Model file for the job. Use its own axes, mm. A direction names the side the tool comes from. Coordinates: 2 decimals unless noted, no trailing zeros. Loops run counter-clockwise (first coordinate to the right, second up) from the corner with the lowest first, then second, coordinate; pieces in that order, holes last. Notation, with made-up numbers: (35.25, 21.25) -> (61.25, 21.25) arc R28 ccw to (61.25, 50.25) -> close; hole circle Ø1 at (-18, 25). An arc over 180 degrees is marked (long way). Use one line per item in the form item = value.
```python
from build123d import *

# Parameters (mm, degrees)
PAD_DEPTH               = 1
PAD001_DEPTH            = 3
PAD002_DEPTH            = 5
PAD_MIRRORED_2_DEPTH    = 1
PAD001_MIRRORED_2_DEPTH = 3
PAD002_MIRRORED_2_DEPTH = 5


with BuildPart() as part:
    # Sketch → Pad (new body)
    with BuildSketch(Plane.XY):
        with BuildLine():
            Line((0, 0), (19.5, 0))
            Line((19.5, 0), (19.5, 28.5))
            Line((19.5, 28.5), (0, 28.5))
            Line((0, 28.5), (0, 23.2))
            ThreePointArc((0, 18.8), (2.2, 21), (0, 23.2))
            Line((0, 18.8), (0, 0))
        make_face()
    pad = extrude(amount=PAD_DEPTH)

    # Sketch001 → Pad001 (join)
    with BuildSketch(Plane.XY):
        with BuildLine():
            ThreePointArc((0, 18.8), (2.2, 21), (0, 23.2))
            Line((0, 23.2), (0, 26.2))
            ThreePointArc((0, 15.8), (5.2, 21), (0, 26.2))
            Line((0, 18.8), (0, 15.8))
        make_face()
    pad001 = extrude(amount=PAD001_DEPTH)

    # Sketch002 → Pad002 (join)
    with BuildSketch(Plane.XY):
        with BuildLine():
            Line((19.5, 0), (19.5, 28.5))
            Line((19.5, 28.5), (0, 28.5))
            Line((0, 28.5), (0, 31.5))
            Line((0, 31.5), (19.5, 31.5))
            ThreePointArc((22.5, 28.5), (21.62132, 30.62132), (19.5, 31.5))
            Line((22.5, 0), (22.5, 28.5))
            Line((19.5, 0), (22.5, 0))
        make_face()
    pad002 = extrude(amount=PAD002_DEPTH)

    # Sketch Mirrored 2 → Pad Mirrored 2 (add)
    with BuildSketch(Plane(origin=(0, 0, 0), x_dir=(-1, 0, 0), z_dir=(0, 0, -1))):
        with BuildLine():
            Line((0, 0), (19.5, 0))
            Line((19.5, 0), (19.5, 28.5))
            Line((19.5, 28.5), (0, 28.5))
            Line((0, 28.5), (0, 23.2))
            ThreePointArc((0, 18.8), (2.2, 21), (0, 23.2))
            Line((0, 18.8), (0, 0))
        make_face()
    pad_mirrored_2 = extrude(amount=-PAD_MIRRORED_2_DEPTH)

    # Sketch001 Mirrored 2 → Pad001 Mirrored 2 (add)
    with BuildSketch(Plane(origin=(0, 0, 0), x_dir=(-1, 0, 0), z_dir=(0, 0, -1))):
        with BuildLine():
            ThreePointArc((0, 18.8), (2.2, 21), (0, 23.2))
            Line((0, 23.2), (0, 26.2))
            ThreePointArc((0, 15.8), (5.2, 21), (0, 26.2))
            Line((0, 18.8), (0, 15.8))
        make_face()
    pad001_mirrored_2 = extrude(amount=-PAD001_MIRRORED_2_DEPTH)

    # Sketch002 Mirrored 2 → Pad002 Mirrored 2 (add)
    with BuildSketch(Plane(origin=(0, 0, 0), x_dir=(-1, 0, 0), z_dir=(0, 0, -1))):
        with BuildLine():
            Line((19.5, 0), (19.5, 28.5))
            Line((19.5, 28.5), (0, 28.5))
            Line((0, 28.5), (0, 31.5))
            Line((0, 31.5), (19.5, 31.5))
            ThreePointArc((22.5, 28.5), (21.62132, 30.62132), (19.5, 31.5))
            Line((22.5, 0), (22.5, 28.5))
            Line((19.5, 0), (22.5, 0))
        make_face()
    pad002_mirrored_2 = extrude(amount=-PAD002_MIRRORED_2_DEPTH)

    # Mirrored001: Pad, Pad001, Pad002, Pad Mirrored 2, Pad001 Mirrored 2, Pad002 Mirrored 2 across Sketch H_Axis
    add(pad.mirror(Plane.ZX))
    add(pad001.mirror(Plane.ZX))
    add(pad002.mirror(Plane.ZX))
    add(pad_mirrored_2.mirror(Plane.ZX))
    add(pad001_mirrored_2.mirror(Plane.ZX))
    add(pad002_mirrored_2.mirror(Plane.ZX))


solid = part.part
```
Q1. Wall check: line 1 along X through (y, z) = (-21, 1.25); line 2 along X through (y, z) = (14, 1.7); line 3 along Y through (x, z) = (-6, 2.05). Give the ranges that are in metal, low to high.
Result:
line_1 = -22.5 to -19.5, -5.2 to -2.2, 2.2 to 5.2, 19.5 to 22.5
line_2 = -22.5 to -19.5, 19.5 to 22.5
line_3 = -31.5 to -28.5, 28.5 to 31.5
Q2. Band-saw the part on D-D, the plane z = 3.95. Write the cut outline in (x, y).
Result:
outline = (-22.5, -28.5) arc R3 ccw to (-19.5, -31.5) -> (19.5, -31.5) arc R3 ccw to (22.5, -28.5) -> (22.5, 28.5) arc R3 ccw to (19.5, 31.5) -> (-19.5, 31.5) arc R3 ccw to (-22.5, 28.5) -> close; hole (-19.5, -28.5) -> (19.5, -28.5) -> (19.5, 28.5) -> (-19.5, 28.5) -> close
Q3. Band-saw the part on C-C, the plane y = 21. Write the cut outline in (x, z).
Result:
outline = (-22.5, 0) -> (-2.2, 0) -> (-2.2, 3) -> (-5.2, 3) -> (-5.2, 1) -> (-19.5, 1) -> (-19.5, 5) -> (-22.5, 5) -> close; (2.2, 0) -> (22.5, 0) -> (22.5, 5) -> (19.5, 5) -> (19.5, 1) -> (5.2, 1) -> (5.2, 3) -> (2.2, 3) -> close
Q4. Band-saw the part on B-B, the plane y = 8. Write the cut outline in (x, z), and give its area (3 significant figures).
Result:
outline = (-22.5, 0) -> (22.5, 0) -> (22.5, 5) -> (19.5, 5) -> (19.5, 1) -> (-19.5, 1) -> (-19.5, 5) -> (-22.5, 5) -> close
area = 69.0 mm2
Q5. Mould opens along Y. For faces 1 (the face through (-20, 0, 5)), 2 (the face through (-1.56, 16.04, 1.99)), 3 (the face through (0, 31.5, 2)), 4 (the face through (1.56, -16.04, 1.99)) say: released by +Y, released by -Y, zero draft, split by the parting line, or undercut.
Result:
face_1 = zero draft
face_2 = undercut
face_3 = released by +Y
face_4 = undercut
Q6. Which spindle directions (+Z, -Z, +X, -X, +Y, -Y) get a long thin tool onto all of the face, cutting with end or side? Do faces 5 (the face through (-22.5, 0, 2)), 6 (the face through (0, 28.5, 3)). Say none if no direction does.
Result:
face_5 = +Z, -Z, -X, +Y, -Y
face_6 = +Z
Q7. Pin check, flat tips, straight feed: pin 1 Ø11.5 at (x, y) = (-1.5, -9.5) entering from +Z; pin 2 Ø1.5 at (x, y) = (-15.5, -18) entering from -Z; pin 3 Ø3.5 at (x, y) = (0, -21) entering from +Z; pin 4 Ø5 at (x, y) = (0, 23.5) entering from +Z. Stop position of each tip, or through.
Result:
pin_1 = 1
pin_2 = 0
pin_3 = through
pin_4 = 3
Q8. Band-saw the part on A-A, the plane x = 0. Write the cut outline in (y, z).
Result:
outline = (-31.5, 0) -> (-23.2, 0) -> (-23.2, 3) -> (-26.2, 3) -> (-26.2, 1) -> (-28.5, 1) -> (-28.5, 5) -> (-31.5, 5) -> close; (-18.8, 0) -> (18.8, 0) -> (18.8, 3) -> (15.8, 3) -> (15.8, 1) -> (-15.8, 1) -> (-15.8, 3) -> (-18.8, 3) -> close; (23.2, 0) -> (31.5, 0) -> (31.5, 5) -> (28.5, 5) -> (28.5, 1) -> (26.2, 1) -> (26.2, 3) -> (23.2, 3) -> close
